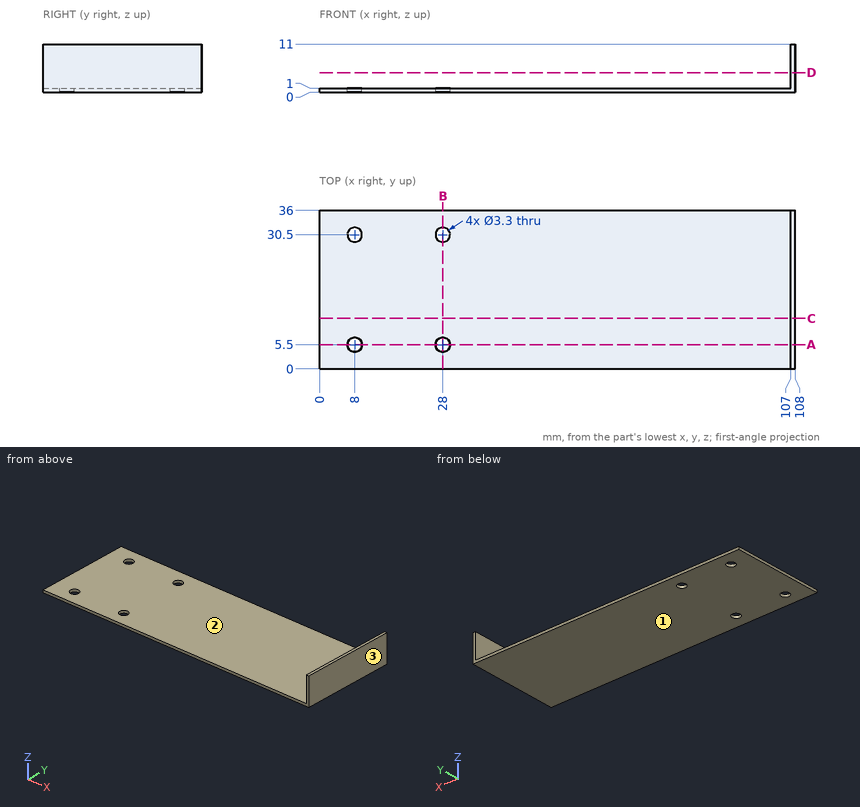
Print and shaded views of the part. All mm, measured from the part's lowest x, y and z. Round coordinates to 2 decimals unless told otherwise and drop trailing zeros. Write each loop counter-clockwise with the first axis right and the second up, starting at its lowest first coordinate (ties: lowest second). Pieces come first, ordered by that corner, then holes.
(1) Slice it at B-B, the plane x = 28. Write the cut outline in (y, z), and give its area (3 significant figures).
(2) Slice it at A-A, the plane y = 5.5. Write the cut outline in (x, z), and give its area (3 significant figures).
(3) Mould opens along Z. For the marked faces 1, 2 and 3 say: pulls with the +Z half, pulls with the -Z half, needs draft (parallel to the pull), parting line crosses it, or undercut.
(4) Drop flat-ended pins along their axis: P1, Ø5.5, axis at x = 8, y = 5.5, coming from the +Z side; P2, Ø6, axis at x = 66, y = 8, coming from the -Z side; P3, Ø5, axis at y = 25, z = 5, coming from the -X side. Give the stop position or say it passes through.
(5) Slice it at C-C, the plane y = 11.5. Write the cut outline in (x, z).
(6) Slice it at D-D, the plane z = 4.5. Write the cut outline in (x, y), and give its area (3 significant figures).
(7) Probe line 1 along X through (y, z) = (5.5, 0.55); line 2 along Y through (x, z) = (8, 0.65); line 3 along X through (y, z) = (31.5, 3.75). List the from-to ranges inside material, lowest first.
From the geometry:
1. outline: (0, 0) - (3.85, 0) - (3.85, 1) - (0, 1) - close; (7.15, 0) - (28.85, 0) - (28.85, 1) - (7.15, 1) - close; (32.15, 0) - (36, 0) - (36, 1) - (32.15, 1) - close
1. area: 29.4 mm2
2. outline: (0, 0) - (6.35, 0) - (6.35, 1) - (0, 1) - close; (9.65, 0) - (26.35, 0) - (26.35, 1) - (9.65, 1) - close; (29.65, 0) - (108, 0) - (108, 11) - (107, 11) - (107, 1) - (29.65, 1) - close
2. area: 111 mm2
3. face 1: pulls with the -Z half
3. face 2: pulls with the +Z half
3. face 3: needs draft
4. P1: stops at z = 1
4. P2: stops at z = 0
4. P3: stops at x = 107
5. outline: (0, 0) - (108, 0) - (108, 11) - (107, 11) - (107, 1) - (0, 1) - close
6. outline: (107, 0) - (108, 0) - (108, 36) - (107, 36) - close
6. area: 36.0 mm2
7. line 1: x = 0 to 6.35, 9.65 to 26.35, 29.65 to 108
7. line 2: y = 0 to 3.85, 7.15 to 28.85, 32.15 to 36
7. line 3: x = 107 to 108
